Autodesk Inventor part; units mm, degrees
ref_plane "YZ Plane" through (0, 0, 0) normal (1, 0, 0) x (0, 1, 0)
ref_plane "XZ Plane" through (0, 0, 0) normal (0, 1, 0) x (-1, 0, 0)
ref_plane "XY Plane" through (0, 0, 0) normal (0, 0, 1) x (1, 0, 0)
sketch "Esboço1" plane through (0, 0, 0) normal (0, 1, 0) x (-1, 0, 0)
  circle A0 centre (0, 0) radius 18
  dimension "d0" = 36
extrude "Extrusão1" add sketch "Esboço1" along normal blind 15
sketch "Esboço2" plane through (0, 15, 0) normal (0, 1, 0) x (1, 0, 0)
  circle A0 centre (0, 0) radius 5
  dimension "d3" = 10
extrude "Extrusão2" add sketch "Esboço2" along normal blind 70
thread "Rosca1"
chamfer "Chamfer1" distance 0.5 angle 45 1 edges at (18, 0, 0)
chamfer "Chamfer2" distance 0.5 angle 45 1 edges at (18, 15, 0)
equation "\"Raio_vergadura\" = Espessura"
equation "\"Largura_alívio_de_vergadura\" = Espessura"
equation "\"Profundidade_alívio_de_vergadura\" = 0.5 * Espessura"
equation "\"Tamanho_alívio_de_dobra\" = 4 * Espessura"
equation "\"Remanescente_mínimo\" = 2 * Espessura"
equation "\"Raiodetransição\" = Raio_vergadura"
equation "\"Tamanho_de_raio_de_Jacobi\" = Raio_vergadura"
equation "\"TamanhoFolga\" = Espessura"
properties part number "Probe" material "Aluminum 6061"
Part model, mm, in its own coordinate system. A direction names the side the tool comes from. Coordinates: 2 decimals unless noted, no trailing zeros. Loops run counter-clockwise (first coordinate to the right, second up) from the corner with the lowest first, then second, coordinate; pieces in that order, holes last. Notation, with made-up numbers: M 52.25,-21.5 L 76.25,-21.5 A24 cw 76.25,3.5 Z; hole C -4.5,76 d10. An arc over 180 degrees is marked long. Use a Markdown table: item, result. Add a question column.
Q1. Cut at D-D (y = 76). Write the cut outline in (x, z), and give its area (3 significant figures).
Q2. Pin check, flat tips, straight feed: P1, Ø6, axis at x = 7.5, y = 13.5, coming from the +Z side; P2, Ø10, axis at x = 6, y = 9.5, coming from the -Z side; P3, Ø12, axis at x = 11.5, z = 10, coming from the +Y side. Stop position of each tip, or through.
Q3. Cut at B-B (x = 0). Write the cut outline in (y, z), and give its area (3 significant figures).
Q4. Probe L1, parallel to Y at x = -13, z = -7; L2, parallel to Z at x = 12.5, y = 14.5; L3, parallel to Z at x = 5.5, y = 8.5. List the from-to ranges inside material, lowest first.
Q5. Cut at C-C (y = 7). Write the cut outline in (x, z).
Q6. Which spindle directions (+Z, -Z, +X, -X, +Y, -Y) get a long thin tool onto all of the face, cutting with end or side? Do faces 1 (the cylindrical face through (-1.08, 49.51, -4.88)), 2 (the cylindrical face through (2.343, 7.402, -17.847)). Say none if no direction does.
Q7. Cut at A-A (z = 0). Write the cut outline in (x, y).
Worked out:
| question | item | result |
|---|---|---|
| 1 | outline | C 0,0 d10 |
| 1 | area | 78.5 mm2 |
| 2 | P1 | stops at z = 17.43 |
| 2 | P2 | stops at z = -17.97 |
| 2 | P3 | stops at y = 15 |
| 3 | outline | M 0,-17.5 L 0.5,-18 L 14.5,-18 L 15,-17.5 L 15,-5 L 85,-5 L 85,5 L 15,5 L 15,17.5 L 14.5,18 L 0.5,18 L 0,17.5 Z |
| 3 | area | 1,240 mm2 |
| 4 | L1 | y = 0 to 15 |
| 4 | L2 | z = -12.95 to 12.95 |
| 4 | L3 | z = -17.14 to 17.14 |
| 5 | outline | C 0,0 d36 |
| 6 | face 1 | +Y |
| 6 | face 2 | +Y, -Y |
| 7 | outline | M -18,0.5 L -17.5,0 L 17.5,0 L 18,0.5 L 18,14.5 L 17.5,15 L 5,15 L 5,85 L -5,85 L -5,15 L -17.5,15 L -18,14.5 Z |
